from build123d import *

# Parameters (mm, degrees)
SKETCH_1_R      = 11
SKETCH_1_R_2    = 10
EXTRUDE_1_DEPTH = 60
EXTRUDE_START   = -10
SKETCH_2_R      = 16
SKETCH_2_R_2    = 11
EXTRUDE_3_DEPTH = 2
SKETCH_3_R      = 16
SKETCH_3_R_2    = 11
EXTRUDE_4_DEPTH = 2


with BuildPart() as part:
    # Эскиз1 → Бобышка-Вытянуть1 (new body)
    with BuildSketch(Plane(origin=(0, 0, 0), x_dir=(1, 0, 0), z_dir=(0, 1, 0))):
        Circle(SKETCH_1_R)
        Circle(SKETCH_1_R_2, mode=Mode.SUBTRACT)
    extrude(amount=EXTRUDE_1_DEPTH)

    # Эскиз2 → Бобышка-Вытянуть3 (add)
    with BuildSketch(Plane(origin=(0, 60, 0), x_dir=(1, 0, 0), z_dir=(0, 1, 0)).offset(EXTRUDE_START)):
        Circle(SKETCH_2_R)
        Circle(SKETCH_2_R_2, mode=Mode.SUBTRACT)
    extrude(amount=-EXTRUDE_3_DEPTH)

    # Эскиз3 → Бобышка-Вытянуть4 (add)
    with BuildSketch(Plane.XZ.offset(EXTRUDE_START)):
        Circle(SKETCH_3_R)
        Circle(SKETCH_3_R_2, mode=Mode.SUBTRACT)
    extrude(amount=-EXTRUDE_4_DEPTH)


solid = part.part
Geometry check sheet. Reference: the model listing, model coordinates, mm. A direction names the side the tool comes from. Give positions to 0.01 mm unless a question says otherwise; leave off trailing zeros. Order: outer loops, then holes, each group sorted by start corner. A loop starts at its lowest first (then second) coordinate and runs counter-clockwise, first axis right, second up. Notation, with made-up numbers: (-5.5, 3.5) - (25.5, 3.5) arc R10 cw to (25.5, 22.5) - close; hole circle Ø1 at (-20.5, 76.25). An arc over 180 degrees is marked (long way). Answer as a JSON object with one key per item and string values.
(1) Tool access check on faces 4 (the flat face through (3, 50, -11)), 5 (the flat face through (3, 12, 11)), 6 (the cylindrical face through (-3.47, 49.01, 15.62)), 7 (the flat face through (3, 10, 11)). Record the directions out of +Z, -Z, +X, -X, +Y, -Y that give a thin tool (end or side, any length) a straight path to the whole face; none if there is none.
Report:
{"face 4": "+Y", "face 5": "none", "face 6": "+Y, -Y", "face 7": "-Y"}
(2) Draft check along X on faces 1 (the flat face through (2, 0, 10)), 2 (the cylindrical face through (-2.17, 29.58, 9.76)), 3 (the cylindrical face through (-2.38, 54.93, 10.74)). Enter one of: released by +X, released by -X, zero draft, split by the parting line, or undercut.
Report:
{"face 1": "zero draft", "face 2": "undercut", "face 3": "split by the parting line"}
(3) Depth check by flat-ended pin: pin 1 Ø8 at (x, y) = (10, 39.5) entering from +Z; pin 2 Ø1 at (x, z) = (9, 10) entering from +Y; pin 3 Ø8 at (x, z) = (-2, -1) entering from -Y; pin 4 Ø5 at (x, y) = (4.5, 10.5) entering from +Z. Enter the tip coordinate at first touch or a pass-through.
Report:
{"pin 1": "z = 9.22", "pin 2": "y = 50", "pin 3": "through", "pin 4": "z = 15.87"}
(4) Cross-section at A-A (z = 0). Record the cut outline in (x, y), then the cut area to 3 significant figures.
Report:
{"outline": "(-16, 10) - (-11, 10) - (-11, 0) - (-10, 0) - (-10, 60) - (-11, 60) - (-11, 50) - (-16, 50) - (-16, 48) - (-11, 48) - (-11, 12) - (-16, 12) - close; (10, 0) - (11, 0) - (11, 10) - (16, 10) - (16, 12) - (11, 12) - (11, 48) - (16, 48) - (16, 50) - (11, 50) - (11, 60) - (10, 60) - close", "area": "160 mm^2"}
(5) Material ranges on line 1 (Y direction, x = 4, z = 13.5); line 2 (X direction, y = 27, z = 0), recorded low to high.
Report:
{"line 1": "10 to 12, 48 to 50", "line 2": "-11 to -10, 10 to 11"}
(6) Cross-section at B-B (x = 0). Record the cut outline in (y, z), then the cut area to 3 significant figures.
Report:
{"outline": "(0, -11) - (10, -11) - (10, -16) - (12, -16) - (12, -11) - (48, -11) - (48, -16) - (50, -16) - (50, -11) - (60, -11) - (60, -10) - (0, -10) - close; (0, 10) - (60, 10) - (60, 11) - (50, 11) - (50, 16) - (48, 16) - (48, 11) - (12, 11) - (12, 16) - (10, 16) - (10, 11) - (0, 11) - close", "area": "160 mm^2"}
(7) Cross-section at D-D (x = 12.5). Record the cut outline in (y, z), then the cut area to 3 significant figures.
Report:
{"outline": "(10, -9.99) - (12, -9.99) - (12, 9.99) - (10, 9.99) - close; (48, -9.99) - (50, -9.99) - (50, 9.99) - (48, 9.99) - close", "area": "79.9 mm^2"}
(8) Cross-section at C-C (y = 17). Record the cut outline in (x, z).
Report:
{"outline": "circle Ø22 at (0, 0); hole circle Ø20 at (0, 0)"}
